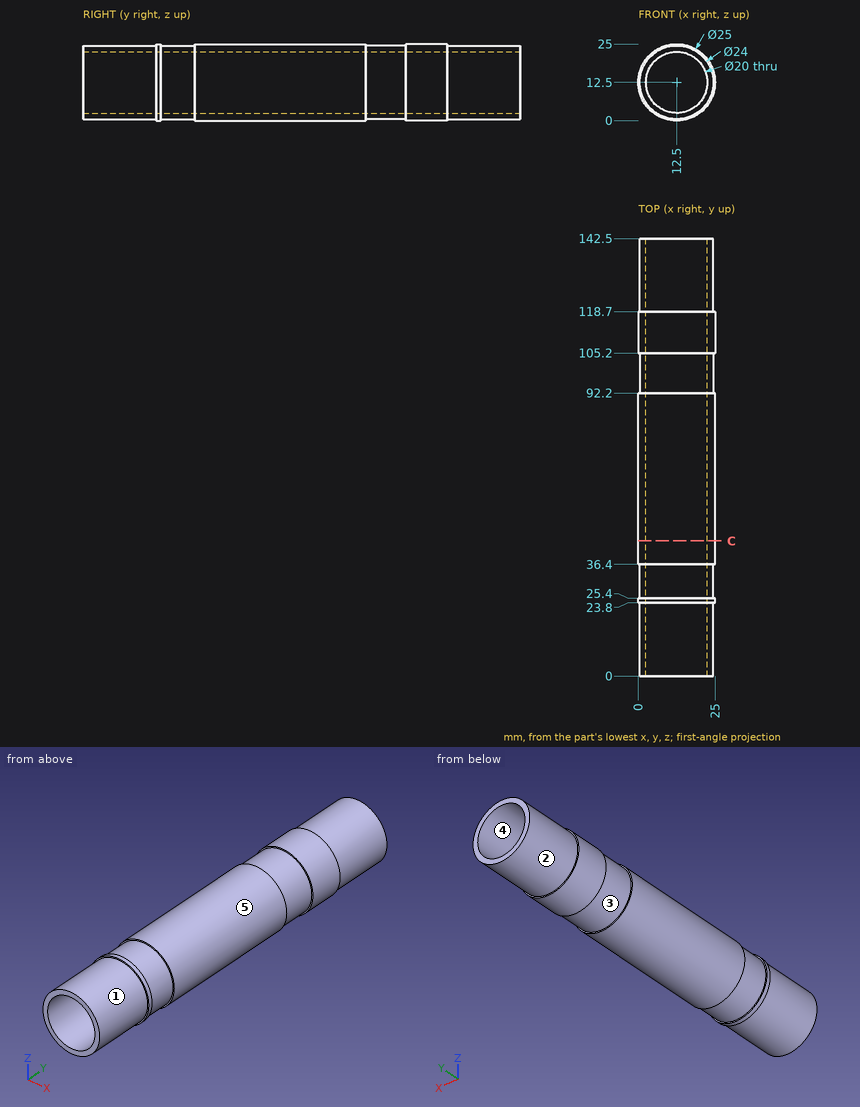
The figure shows three views and two pictorial views of one solid part (mm, origin at its lowest corner). Answer the questions. A direction names the side the tool comes from. Coordinates: 2 decimals unless noted, no trailing zeros. Loops run counter-clockwise (first coordinate to the right, second up) from the corner with the lowest first, then second, coordinate; pieces in that order, holes last.
1) Find section C-C on y = 44. Write down the section's boundary in (x, z), then the cut area to 3 significant figures.
2) Find the intervals of material crossed by L1, parallel to Z at x = 12.5, y = 65.5; L2, parallel to Z at x = 12.5, y = 93, in increasing order.
3) Flat-ended cylindrical pins translate along their axes: pin 1 Ø10 at (x, z) = (13.5, 19.5) entering from +Y; pin 2 Ø10 at (y, z) = (107, 2.5) entering from -X; pin 3 Ø4 at (x, y) = (4, 32.5) entering from +Z; pin 4 Ø1 at (y, z) = (105.5, 9) entering from +X. Find the tip coordinate at first contact, or state that the pin passes through.
4) Determine the mould class of the marked faces 4 and 5 for opening direction X: pulls with the +X half, pulls with the -X half, needs draft (parallel to the pull), parting line crosses it, or undercut.
5) A tool of negligible diameter and unlimited length cuts with its end or side. For the marked faces 1, 2 and 3, from which of +Z, -Z, +X, -X, +Y, -Y can it reach the whole face along a straight path? Write none if from no direction.
Values:
1. outline: circle Ø25 at (12.5, 12.5); hole circle Ø20 at (12.5, 12.5)
1. area: 177 mm2
2. L1: z = 0 to 2.5, 22.5 to 25
2. L2: z = 0.5 to 2.5, 22.5 to 24.5
3. pin 1: stops at y = 142.5
3. pin 2: stops at x = 1.04
3. pin 3: stops at z = 22.59
3. pin 4: stops at x = 24.63
4. face 4: undercut
4. face 5: parting line crosses it
5. face 1: -Y
5. face 2: +Y
5. face 3: none
